```python
from build123d import *

# Parameters (mm, degrees)
BOSS_EXTRUDE1_DEPTH = 1.524


with BuildPart() as part:
    # Sketch1 → Boss-Extrude1 (new body)
    with BuildSketch(Plane.XY):
        with BuildLine():
            Line((47.381308576, -13.076354562), (55.343944742, -14.432422978))
            ThreePointArc((55.343944742, -14.432422978), (55.855819335, -14.328185498), (56.163893215, -13.906318771))
            ThreePointArc((56.163893215, -13.906318771), (55.680504041, -11.077688455), (53.220198686, -9.600626466))
            Line((53.220198686, -9.600626466), (45.266067061, -8.034115775))
            ThreePointArc((45.266067061, -8.034115775), (40.237375781, -4.755718158), (36.574211612, 0))
            ThreePointArc((36.574211612, 0), (35.55871494, -5.254533576), (36.018806888, -10.586481811))
            ThreePointArc((36.018806888, -10.586481811), (35.025995436, -11.496620285), (33.780750037, -12.009836144))
            ThreePointArc((33.780750037, -12.009836144), (29.778374213, -13.039276401), (25.669954537, -12.592457382))
            ThreePointArc((25.669954537, -12.592457382), (26.366552456, -13.076757004), (26.920206789, -13.719611314))
            ThreePointArc((26.920206789, -13.719611314), (22.157152762, -15.15851527), (17.456411215, -16.789514096))
            ThreePointArc((17.456411215, -16.789514096), (12.832168531, -18.332197491), (7.980688074, -18.808254041))
            ThreePointArc((7.980688074, -18.808254041), (8.253415585, -19.676221582), (8.349810899, -20.580907104))
            ThreePointArc((8.349810899, -20.580907104), (6.937406163, -21.247776917), (5.53361242, -21.932587557))
            ThreePointArc((5.53361242, -21.932587557), (3.944680946, -21.988663657), (2.853783543, -20.83203467))
            ThreePointArc((2.853783543, -20.83203467), (2.29585657, -19.263543096), (1.704966772, -17.707169885))
            ThreePointArc((1.704966772, -17.707169885), (1.284069131, -14.122482995), (0.560307739, -10.586481811))
            ThreePointArc((0.560307739, -10.586481811), (0.415674848, -11.924982959), (-0.282069682, -13.076354562))
            ThreePointArc((-0.282069682, -13.076354562), (-3.357054523, -7.162746337), (-6.920105474, -1.52972211))
            ThreePointArc((-6.920105474, -1.52972211), (-8.0910802, 1.949544484), (-9.710699696, 5.243980782))
            ThreePointArc((-9.710699696, 5.243980782), (-9.857305852, 4.075018277), (-10.290972629, 2.979618885))
            ThreePointArc((-10.290972629, 2.979618885), (-13.777130717, 7.023766683), (-17.528779794, 10.822919067))
            ThreePointArc((-17.528779794, 10.822919067), (-21.284368064, 16.919530678), (-26.897153204, 21.365850433))
            ThreePointArc((-26.897153204, 21.365850433), (-25.887369361, 19.461878078), (-25.598425379, 17.326161451))
            ThreePointArc((-25.598425379, 17.326161451), (-39.347249709, 24.806966458), (-54.370546376, 29.199365714))
            ThreePointArc((-54.370546376, 29.199365714), (-61.003451809, 29.476578966), (-67.319072822, 31.522358252))
            ThreePointArc((-67.319072822, 31.522358252), (-61.733688319, 27.51480849), (-55.009920851, 26.08375078))
            ThreePointArc((-55.009920851, 26.08375078), (-52.038783927, 25.331807522), (-49.101103933, 24.458246116))
            ThreePointArc((-49.101103933, 24.458246116), (-50.963404132, 24.042209603), (-52.230913262, 22.615791355))
            ThreePointArc((-52.230913262, 22.615791355), (-47.957226248, 23.275149282), (-43.703205331, 22.498966559))
            ThreePointArc((-43.703205331, 22.498966559), (-34.98884104, 18.269729883), (-26.897153204, 12.945147661))
            ThreePointArc((-26.897153204, 12.945147661), (-28.611374467, 12.792404738), (-30.222607976, 12.187581193))
            ThreePointArc((-30.222607976, 12.187581193), (-26.225509878, 11.251375507), (-22.559534857, 9.403700904))
            ThreePointArc((-22.559534857, 9.403700904), (-19.030321473, 6.083870505), (-15.72447016, 2.541559382))
            ThreePointArc((-15.72447016, 2.541559382), (-13.836348231, -0.215104475), (-12.02203426, -3.020895781))
            ThreePointArc((-12.02203426, -3.020895781), (-13.508524403, -3.175087526), (-14.995014547, -3.020895781))
            ThreePointArc((-14.995014547, -3.020895781), (-11.58739515, -5.203150516), (-8.916043995, -8.242556493))
            ThreePointArc((-8.916043995, -8.242556493), (-5.974041698, -13.791075709), (-3.312350182, -19.479383127))
            ThreePointArc((-3.312350182, -19.479383127), (-4.870972445, -19.369578502), (-6.329147764, -18.808254041))
            ThreePointArc((-6.329147764, -18.808254041), (-3.312350182, -21.839623943), (-0.906453557, -25.375431145))
            ThreePointArc((-0.906453557, -25.375431145), (-0.657734758, -26.037552601), (-0.412739096, -26.701060692))
            ThreePointArc((-0.412739096, -26.701060692), (1.91016195, -29.006645717), (5.168319653, -28.696807117))
            ThreePointArc((5.168319653, -28.696807117), (6.748763707, -27.788827847), (8.349810899, -26.917692008))
            ThreePointArc((8.349810899, -26.917692008), (8.630214839, -27.78643645), (8.562623992, -28.696807117))
            ThreePointArc((8.562623992, -28.696807117), (10.486664845, -26.455513742), (12.868412887, -24.70834304))
            ThreePointArc((12.868412887, -24.70834304), (16.869160672, -23.03916113), (20.955745156, -21.592793838))
            ThreePointArc((20.955745156, -21.592793838), (21.05258172, -22.797241034), (20.746541516, -23.966176344))
            ThreePointArc((20.746541516, -23.966176344), (23.495531579, -21.764324116), (26.549791209, -20.010300822))
            ThreePointArc((26.549791209, -20.010300822), (29.81474898, -19.288764723), (33.107408372, -18.706563972))
            ThreePointArc((33.107408372, -18.706563972), (34.43330114, -18.558524355), (35.762761976, -18.446984027))
            ThreePointArc((35.762761976, -18.446984027), (35.632573955, -19.733193435), (34.951522192, -20.83203467))
            ThreePointArc((34.951522192, -20.83203467), (38.192011454, -19.210457415), (41.722919829, -18.396228022))
            ThreePointArc((41.722919829, -18.396228022), (45.188062045, -18.704651863), (48.622209673, -19.26049889))
            ThreePointArc((48.622209673, -19.26049889), (48.214896908, -20.366352247), (47.381308576, -21.199386357))
            ThreePointArc((47.381308576, -21.199386357), (50.647879824, -20.381891812), (53.469866719, -18.544726873))
            ThreePointArc((53.469866719, -18.544726873), (54.428390669, -17.883217687), (55.261101332, -17.068996882))
            ThreePointArc((55.261101332, -17.068996882), (55.403709497, -16.34876081), (54.842730354, -15.875073687))
            Line((54.842730354, -15.875073687), (47.128232405, -14.561068095))
            Line((47.128232405, -14.561068095), (47.381308576, -13.076354562))
        make_face()
    extrude(amount=BOSS_EXTRUDE1_DEPTH)


solid = part.part
```
Geometry check sheet. Reference: the model listing, model coordinates, mm. A direction names the side the tool comes from. Coordinates: 2 decimals unless noted, no trailing zeros. Order: outer loops, then holes, each group sorted by start corner. A loop starts at its lowest first (then second) coordinate and runs counter-clockwise, first axis right, second up. Notation, with made-up numbers: (55.5, 60.25) - (88.5, 60.25) arc R18 ccw to (88.5, 64.25) - close; hole circle Ø9 at (6, -22.5). An arc over 180 degrees is marked (long way). Answer as a JSON object with one key per item and string values. Group by question number.
Item 1: Sectioned sample at A-A, the plane x = -41. Record the cut outline in (y, z), and give its area (3 significant figures).
Item 2: Draft check along Y on faces 3 (the face through (-21.218, 16.844, 0.751)), 4 (the face through (1.87, -28.99, 0.75)), 5 (the face through (-13.86, -0.18, 0.75)). Enter one of: +Y half, -Y half, draft (parallel to the pull), parting line (faces both ways), or undercut.
Item 3: Sectioned sample at B-B, the plane y = 16. Record the cut outline in (x, z), and give its area (3 significant figures).
Item 4: Scan lines: probe 1 along X at (y, z) = (21, 1.35); probe 2 along Y at (x, z) = (-14, 1.15); probe 3 along X at (y, z) = (-2.5, 0.6). Record each from-to range of solid material in increasing order.
Item 5: Tool access check on faces 1 (the face through (-8.07, 1.9, 0.75)), 2 (the face through (-3.351, -21.793, 0.751)). Record the directions out of +Z, -Z, +X, -X, +Y, -Y that give a thin tool (end or side, any length) a straight path to the whole face; none if there is none.
Resolved:
{
 "1": {"outline": "(21.34, 0) - (25.47, 0) - (25.47, 1.52) - (21.34, 1.52) - close", "area": "6.29 mm^2"},
 "2": {"face 3": "+Y half", "face 4": "-Y half", "face 5": "undercut"},
 "3": {"outline": "(-31.26, 0) - (-20.51, 0) - (-20.51, 1.52) - (-31.26, 1.52) - close", "area": "16.4 mm^2"},
 "4": {"probe 1": "-40.27 to -31.49, -26.63 to -26.25", "probe 2": "-3.52 to -3.16, 0.03 to 7.26", "probe 3": "-12.35 to -6.26, 35.9 to 38.18"},
 "5": {"face 1": "+Z, -Z, +Y", "face 2": "+Z, -Z, -X, -Y"}
}
